from build123d import *

# Parameters (mm, degrees)
SKETCH1_R           = 5
BOSS_EXTRUDE1_DEPTH = 5
SKETCH2_R           = 0.25
CUT_EXTRUDE1_DEPTH  = 6
CIRPATTERN1_COUNT   = 12


with BuildPart() as part:
    # Sketch1 → Boss-Extrude1 (new body)
    with BuildSketch(Plane.XY):
        Circle(SKETCH1_R)
    extrude(amount=BOSS_EXTRUDE1_DEPTH)

    # Sketch2 → Cut-Extrude1 (cut, through all)
    with BuildSketch(Plane.XY.offset(5)):
        with Locations((4, 0)):
            Circle(SKETCH2_R)
    cut_extrude1 = extrude(amount=-CUT_EXTRUDE1_DEPTH, mode=Mode.SUBTRACT)

    # CirPattern1: Cut-Extrude1 ×12 about axis
    cirpattern1_axis = Axis((0, 0, 0), (0, 0, 1))
    for i in range(1, CIRPATTERN1_COUNT):
        add(cut_extrude1.rotate(cirpattern1_axis, i * 360 / CIRPATTERN1_COUNT), mode=Mode.SUBTRACT)


solid = part.part
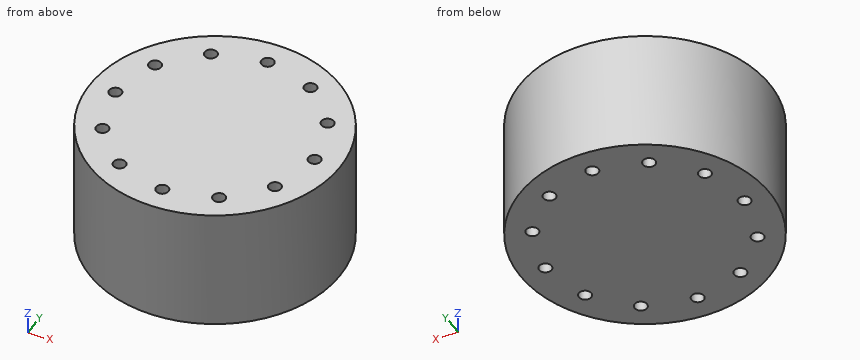
CAD build for the part. Positions are in the model's coordinates, mm. Round coordinates to 2 decimals unless told otherwise and drop trailing zeros. Order: outer loops, then holes, each group sorted by start corner. A loop starts at its lowest first (then second) coordinate and runs counter-clockwise, first axis right, second up. Notation, with made-up numbers: M 87,63.25 L 127,63.25 A12 ccw 127,82.25 Z; hole C -12.5,-31 d5. An arc over 180 degrees is marked long. Use one line per item in the form item = value.
Q1. Saw through at A-A on y = 4. Give the cut face in (x, z), then the cut area to 3 significant figures.
Recorded:
outline = M -3,0 L -0.25,0 L -0.25,5 L -3,5 Z; M 0.25,0 L 3,0 L 3,5 L 0.25,5 Z
area = 27.5 mm^2
Q2. Probe L1, parallel to Y at x = -2, z = 2.45; L2, parallel to Y at x = -4, z = 2.5. List the from-to ranges inside material, lowest first.
Recorded:
L1 = -4.58 to -3.71, -3.21 to 3.21, 3.71 to 4.58
L2 = -3 to -0.25, 0.25 to 3
Q3. Saw through at D-D on y = 2. Give the cut face in (x, z), then the cut area to 3 significant figures.
Recorded:
outline = M -4.58,0 L -3.71,0 L -3.71,5 L -4.58,5 Z; M -3.21,0 L 3.21,0 L 3.21,5 L -3.21,5 Z; M 3.71,0 L 4.58,0 L 4.58,5 L 3.71,5 Z
area = 40.8 mm^2
Q4. Saw through at C-C on x = 0. Give the cut face in (y, z).
Recorded:
outline = M -5,0 L -4.25,0 L -4.25,5 L -5,5 Z; M -3.75,0 L 3.75,0 L 3.75,5 L -3.75,5 Z; M 4.25,0 L 5,0 L 5,5 L 4.25,5 Z
Q5. Flat gauge pins, fed straight in: P1, Ø6, axis at x = 4, y = -4, coming from the +Z side; P2, Ø1, axis at y = -2, z = 2, coming from the -X side; P3, Ø1, axis at x = 1, z = 3, coming from the -Y side. Where does each tip first touch, or does it go through?
Recorded:
P1 = 5
P2 = -4.77
P3 = -4.97
